```python
from build123d import *

# Parameters (mm, degrees)
SKETCH_1_R               = 3.5
EXTRUDE_1_DEPTH          = 2.6
SKETCH_2_R               = 2
EXTRUDE_2_DEPTH          = 8
CHAMFER_1_SIZE           = 0.5
CUT_EXTRUDE_1_DEPTH      = 10.407443861
CUT_EXTRUDE_1_DEPTH_BACK = 10.407443861
SKETCH_3_W               = 1.3
SKETCH_3_H               = 1.2


with BuildPart() as part:
    # Эскиз1 → Бобышка-Вытянуть1 (new body)
    with BuildSketch(Plane.XY):
        Circle(SKETCH_1_R)
    extrude(amount=EXTRUDE_1_DEPTH)

    # Эскиз2 → Бобышка-Вытянуть2 (add)
    with BuildSketch(Plane(origin=(0, 0, 0), x_dir=(-1, 0, 0), z_dir=(0, 0, -1))):
        with Locations(Location((0, 0, 0), (0, 0, 180))):
            Circle(SKETCH_2_R)
    extrude(amount=EXTRUDE_2_DEPTH)

    # Фаска1
    chamfer_1_edges = [part.edges().sort_by_distance(p)[0] for p in [
        (-2, 0, -8),
    ]]
    chamfer(chamfer_1_edges, length=CHAMFER_1_SIZE)

    # Эскиз3 → Вырез-Вытянуть1 (cut, two sides: drawn at the far end of the back side and taken through both)
    with BuildSketch(Plane(origin=(0, 0, 0), x_dir=(0, 0, -1), z_dir=(1, 0, 0)).offset(-CUT_EXTRUDE_1_DEPTH_BACK)):
        with Locations((-1.95, 0)):
            Rectangle(SKETCH_3_W, SKETCH_3_H)
    extrude(amount=CUT_EXTRUDE_1_DEPTH + CUT_EXTRUDE_1_DEPTH_BACK, mode=Mode.SUBTRACT)


solid = part.part
```
Geometry: final body of the model. Coordinates: model frame, mm. A direction names the side the tool comes from. Give positions to 0.01 mm unless a question says otherwise; leave off trailing zeros. Order: outer loops, then holes, each group sorted by start corner. A loop starts at its lowest first (then second) coordinate and runs counter-clockwise, first axis right, second up. Notation, with made-up numbers: (-39, -23) -> (-14, -23) arc R19 ccw to (-14, -10) -> close; hole circle Ø1 at (45.25, 1.5). An arc over 180 degrees is marked (long way). Write each question's results on one line, items separated by ' | '. Start each with the question number.
1) Set-up query: faces 1 (the flat face through (0, 0, 1.3)), 2 (the flat face through (0, 2, 2.6)). Return all of +Z, -Z, +X, -X, +Y, -Y with unobstructed straight access to the full face (end or side cutting, diameter ignored); none if empty.
2) Draft query along Y for faces 3 (the flat face through (0, 0.6, 2)), 4 (the flat face through (2, -2, 0)), 5 (the cylindrical face through (0, 2, -4)). Return one class per face: pulls with the +Y half, pulls with the -Y half, needs draft (parallel to the pull), parting line crosses it, or undercut.
3) Line query: line 1 (Z direction, x = 1, y = 0); line 2 (Z direction, x = 1.5, y = -3); line 3 (Y direction, x = 0, z = -0.25). Output: solid intervals per line, ascending. Write a range as from..to.
4) Section C-C (y = 0). Return loops of the section in (x, z).
5) First-contact query: pin 1 (1.5 mm diameter, centred on x = 1.5, z = -1.5, fed in from +Y); pin 2 (1 mm diameter, centred on x = -0.5, y = 1.5, fed in from -Z); pin 3 (2 mm diameter, centred on x = -1, z = -3.5, fed in from +Y). Flat tips, straight axial feed; report the tip coordinate or a pass-through.
6) Section B-B (z = 2.25). Return loops of the section in (x, y).
7) Section D-D (z = -0.75). Return loops of the section in (x, y).
8) Section A-A (x = 0). Return loops of the section in (y, z).
Calculated:
1) face 1: +Z, +X, -X | face 2: +Z, +X, -X, +Y, -Y
2) face 3: undercut | face 4: needs draft | face 5: parting line crosses it
3) line 1: -8..1.3 | line 2: 0..2.6 | line 3: -2..2
4) outline: (-3.5, 0) -> (-2, 0) -> (-2, -7.5) -> (-1.5, -8) -> (1.5, -8) -> (2, -7.5) -> (2, 0) -> (3.5, 0) -> (3.5, 1.3) -> (-3.5, 1.3) -> close
5) pin 1: y = 1.85 | pin 2: z = -8 | pin 3: y = 2
6) outline: (-3.45, -0.6) arc R3.5 ccw to (3.45, -0.6) -> close; (-3.45, 0.6) -> (3.45, 0.6) arc R3.5 ccw to start
7) outline: circle Ø4 at (0, 0)
8) outline: (-3.5, 0) -> (-2, 0) -> (-2, -7.5) -> (-1.5, -8) -> (1.5, -8) -> (2, -7.5) -> (2, 0) -> (3.5, 0) -> (3.5, 2.6) -> (0.6, 2.6) -> (0.6, 1.3) -> (-0.6, 1.3) -> (-0.6, 2.6) -> (-3.5, 2.6) -> close
